from build123d import *

# Parameters (mm, degrees)
F0_R     = 4.4
F0_R_2   = 3.9
F1_DEPTH = 1
F2_DEPTH = 4.4
F3_R     = 0.3


# Not quite as in the source:
# - a feature names something its author has since deleted; it is built from what else it names


with BuildPart() as f1:
    # F0 (on Top) → F1 (new body)
    with BuildSketch(Plane.XY):
        with Locations((-17.6290911883, 6.9914618582)):
            Circle(F0_R)
        with Locations((-17.6290911883, 6.9914618582)):
            Circle(F0_R_2, mode=Mode.SUBTRACT)
        with Locations((-17.6290911883, 6.9914618582)):
            Circle(F0_R_2)
    extrude(amount=F1_DEPTH)

    # F0 (on Top) → F2 (join)
    with BuildSketch(Plane.XY):
        with Locations((-17.6290911883, 6.9914618582)):
            Circle(F0_R_2)
    extrude(amount=F2_DEPTH)

    # F3
    f3_edges = [f1.edges().sort_by_distance(p)[0] for p in [
        (-21.529091, 6.991462, 4.4),
    ]]
    fillet(f3_edges, radius=F3_R)


solid = f1.part
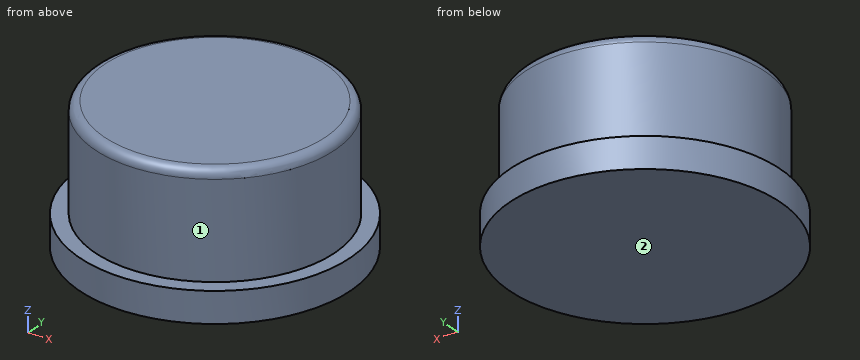
Design review of the part built by this model. Coordinates are the model's own, in mm. Face numbers are marked on the shaded views. A direction names the side the tool comes from. Give positions to 0.01 mm unless a question says otherwise; leave off trailing zeros. Write each loop counter-clockwise with the first axis right and the second up, starting at its lowest first coordinate (ties: lowest second). Pieces come first, ordered by that corner, then holes. Notation, with made-up numbers: M -12.75,-5.75 L 2.25,-5.75 A17 ccw 2.25,27.25 Z; hole C 28.5,68 d7. An arc over 180 degrees is marked long. Return JSON: item names as keys, results as strings. Group by question number.
Item 1: Tool access review of the marked faces 1 and 2: name each direction out of +Z, -Z, +X, -X, +Y, -Y from which nothing blocks a thin tool from reaching the whole face with its end or side.
Item 2: Take a section at B-B (z = 0.5). Give the boundary of the cut face in (x, y).
Item 3: Take a section at A-A (z = 3.7). Give the boundary of the cut face in (x, y), plus the area to 3 significant figures.
Item 4: Wall thickness on line 1 along Z through (x, y) = (-13.75, 6.25); line 2 along Y through (x, z) = (-17.25, 0.55); line 3 along X through (y, z) = (8.75, 3.25): over which ranges is each line inside the solid? List them lowest first.
Return value:
{
 "1": {"face 1": "+Z", "face 2": "-Z, +X, -X, +Y, -Y"},
 "2": {"outline": "C -17.63,6.99 d8.8"},
 "3": {"outline": "C -17.63,6.99 d7.8", "area": "47.8 mm2"},
 "4": {"line 1": "z = 0 to 1", "line 2": "y = 2.61 to 11.38", "line 3": "x = -21.11 to -14.15"}
}
